The listing builds one solid part. Answer for the finished solid, in the listing's coordinates (mm). Face numbers are marked on the shaded views. Coordinates: 2 decimals unless noted, no trailing zeros. Order: outer loops, then holes, each group sorted by start corner. A loop starts at its lowest first (then second) coordinate and runs counter-clockwise, first axis right, second up. Notation, with made-up numbers: (-19.5, 26.5) -> (18.5, 26.5) arc R34 cw to (18.5, 58.5) -> close; hole circle Ø8 at (18.25, -8). An arc over 180 degrees is marked (long way). One line per question, with ' | ' between items.
from build123d import *

# Parameters (mm, degrees)
ESBO_O2_W                  = 8.52075949
ESBO_O2_H                  = 5.764043184
CORTE_EXTRUS_O1_DEPTH      = 21
ESBO_O3_W                  = 2.250213953
ESBO_O3_H                  = 5.764043184
CORTE_EXTRUS_O2_DEPTH      = 21
CORTE_EXTRUS_O2_DEPTH_BACK = 21


with BuildPart() as part:
    # Esboço1 → Revolução1 (revolve)
    with BuildSketch(Plane.XY):
        with BuildLine():
            Line((12.5, 41.646579704), (12.5, 41.506128196))
            add(Edge.make_bspline(
                [(12.5, 41.506128196), (12.338389384, 40.134837747), (12.601764107, 38.305152117), (10.065188923, 35.645635864), (12.500651196, 30.458331587), (16.843058411, 26.670735), (22.76228445, 24.532888043), (24.224821104, 21.349310821), (24.046845434, 19.403944973)],
                knots=[0, 0, 0, 0, 0.101004703, 0.175039834, 0.372875088, 0.603292123, 0.835962091, 1, 1, 1, 1], degree=3))
            ThreePointArc((24.046845434, 19.403944973), (23.264534568, 17.438582109), (22.851836049, 19.513272788))
            add(Edge.make_bspline(
                [(11.308247772, 41.646579704), (11.281760283, 41.421829367), (11.241283492, 40.953310705), (11.207087563, 40.153140867), (11.188443128, 39.325301199), (11.101187915, 38.800994205), (10.999161677, 38.542871248), (10.84650313, 38.269361286), (10.628860527, 37.942340116), (10.368935554, 37.554835556), (10.092298736, 37.083824404), (9.789160953, 36.330082669), (9.651283083, 35.387021367), (9.788883574, 33.919158958), (10.43159292, 32.226529482), (11.534582968, 30.432466838), (12.730902254, 28.915450827), (14.063189235, 27.612944764), (15.516577401, 26.511762273), (17.117458176, 25.575765094), (18.736981448, 24.783206109), (20.230956508, 24.009113027), (21.467011577, 23.176371047), (22.186355151, 22.407246301), (22.575507066, 21.708478748), (22.780108979, 21.111549356), (22.870075885, 20.516676656), (22.88284487, 19.974221941), (22.865553692, 19.663213697), (22.851836049, 19.513272788)],
                knots=[0, 0, 0, 0, 0.015625, 0.03125, 0.0625, 0.09375, 0.109375, 0.125, 0.140625, 0.15625, 0.171875, 0.1875, 0.21875, 0.25, 0.3125, 0.375, 0.4375, 0.5, 0.5625, 0.625, 0.6875, 0.75, 0.8125, 0.875, 0.90625, 0.9375, 0.96875, 0.984375, 1, 1, 1, 1], degree=3))
            add(Edge.make_bspline(
                [(11.308247772, 41.646579704), (10.488228177, 43.241261294), (10.332658745, 45.295831645), (8.575926678, 46.236967031)],
                knots=[0, 0, 0, 0, 1, 1, 1, 1], degree=3))
            Line((8.575926678, 46.236967031), (8.575926678, 55.780385677))
            Line((8.575926678, 55.780385677), (12.5, 55.780385677))
            Line((12.5, 55.780385677), (12.5, 46.236967031))
            Line((12.5, 46.236967031), (12.5, 41.646579704))
        make_face()
    revolve(axis=Axis((0, 44.517371893, 0), (0, -1, 0)))

    # Esboço2 → Corte-extrusão1 (cut)
    with BuildSketch(Plane.XY):
        with Locations((0, 49.017313479)):
            Rectangle(ESBO_O2_W, ESBO_O2_H)
    extrude(amount=-CORTE_EXTRUS_O1_DEPTH, mode=Mode.SUBTRACT)

    # Esboço3 → Corte-extrusão2 (cut, two sides)
    with BuildSketch(Plane(origin=(0, 0, 0), x_dir=(0, 0, -1), z_dir=(1, 0, 0))) as corte_extrus_o2_sk:
        with Locations((11.374893024, 49.017313479)):
            Rectangle(ESBO_O3_W, ESBO_O3_H)
    extrude(amount=CORTE_EXTRUS_O2_DEPTH, mode=Mode.SUBTRACT)
    extrude(corte_extrus_o2_sk.sketch, amount=-CORTE_EXTRUS_O2_DEPTH_BACK, mode=Mode.SUBTRACT)


solid = part.part
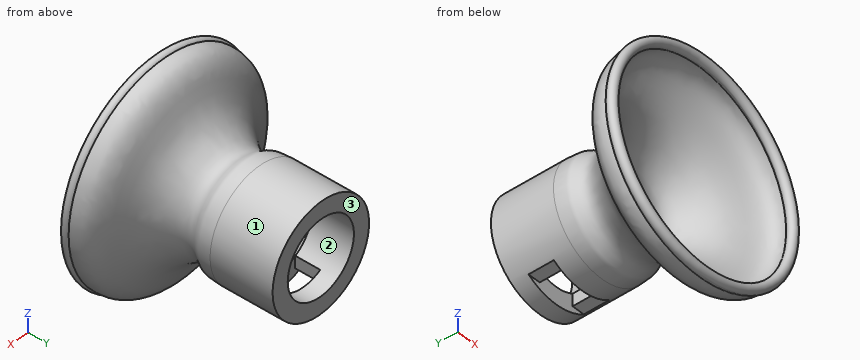
Item 1: Determine the mould class of the marked faces 1, 2 and 3 for opening direction X: pulls with the +X half, pulls with the -X half, needs draft (parallel to the pull), parting line crosses it, or undercut.
Computed values:
face 1: parting line crosses it | face 2: undercut | face 3: needs draft
Item 2: Find the intervals of material crossed by L1, parallel to Y at x = 4.5, z = -10.5; L2, parallel to Z at x = 0, y = 52.5; L3, parallel to Z at x = 0, y = 48.75, in increasing order.
Computed values:
L1: y = 30.66 to 33.1, 36.97 to 46.14, 51.9 to 55.78 | L2: z = -12.5 to -8.58, 8.58 to 12.5 | L3: z = 8.58 to 12.5
Item 3: Section B-B, the plane x = 2.5 is taken. Count the separate pieces of the cut face and the enclosed holes in it, plus the area to 3 significant figures.
Computed values:
separate pieces: 3 | enclosed holes: 0 | area: 152 mm^2
Item 4: Section A-A, the plane y = 50 is taken. Give the vertices of the cut face in (x, z).
Computed values:
outline: (-7.15, -10.25) -> (-4.26, -10.25) -> (-4.26, -7.44) arc R8.58 cw (long way) to (4.26, -7.44) -> (4.26, -10.25) -> (7.15, -10.25) arc R12.5 ccw (long way) to start
Item 5: Each of these flat-tipped pins is pushed along its axis until it touches: pin 1 Ø2 at (y, z) = (32, 1) entering from -X; pin 2 Ø1.5 at (x, z) = (-10.5, -1) entering from -Y; pin 3 Ø1 at (x, z) = (-6.5, -10) entering from -Y. Where does it stop, or does it pass through?
Computed values:
pin 1: stops at x = -12.61 | pin 2: stops at y = 30.85 | pin 3: stops at y = 29.33
